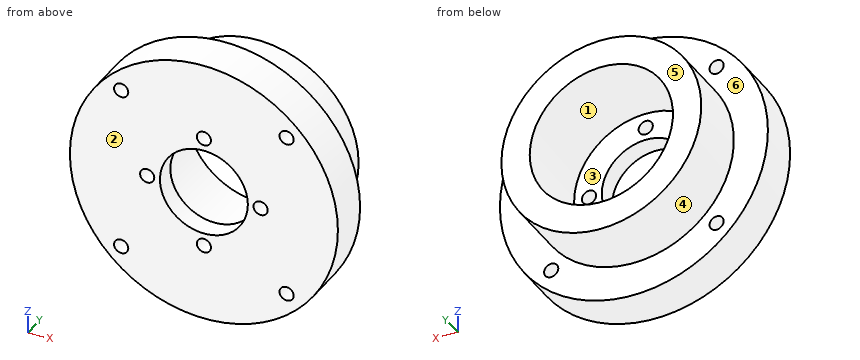
```python
from build123d import *

# Parameters (mm, degrees)
SKETCH1_R           = 35.25
SKETCH1_R_2         = 15.5
BOSS_EXTRUDE1_DEPTH = 7
SKETCH2_R           = 35.25
SKETCH2_R_2         = 25.25
BOSS_EXTRUDE2_DEPTH = 30
SKETCH3_R           = 2.5
CUT_EXTRUDE1_DEPTH  = 7
SKETCH4_R           = 47.25
SKETCH4_R_2         = 35.25
BOSS_EXTRUDE3_DEPTH = 15
SKETCH5_R           = 2.5
CUT_EXTRUDE2_DEPTH  = 15


with BuildPart() as part:
    # Sketch1 → Boss-Extrude1 (new body)
    with BuildSketch(Plane(origin=(0, 0, 0), x_dir=(1, 0, 0), z_dir=(0, 1, 0))):
        Circle(SKETCH1_R)
        Circle(SKETCH1_R_2, mode=Mode.SUBTRACT)
    extrude(amount=BOSS_EXTRUDE1_DEPTH)

    # Sketch2 → Boss-Extrude2 (add)
    with BuildSketch(Plane(origin=(0, 7, 0), x_dir=(1, 0, 0), z_dir=(0, 1, 0))):
        Circle(SKETCH2_R)
        Circle(SKETCH2_R_2, mode=Mode.SUBTRACT)
    extrude(amount=BOSS_EXTRUDE2_DEPTH)

    # Sketch3 → Cut-Extrude1 (cut)
    with BuildSketch(Plane(origin=(0, 7, 0), x_dir=(1, 0, 0), z_dir=(0, 1, 0))):
        with Locations((0, 20)):
            Circle(SKETCH3_R)
        with Locations((20, 0)):
            Circle(SKETCH3_R)
        with Locations((0, -20)):
            Circle(SKETCH3_R)
        with Locations((-20, 0)):
            Circle(SKETCH3_R)
    extrude(amount=-CUT_EXTRUDE1_DEPTH, mode=Mode.SUBTRACT)

    # Sketch4 → Boss-Extrude3 (add)
    with BuildSketch(Plane.XZ):
        Circle(SKETCH4_R)
        Circle(SKETCH4_R_2, mode=Mode.SUBTRACT)
    extrude(amount=-BOSS_EXTRUDE3_DEPTH)

    # Sketch5 → Cut-Extrude2 (cut)
    with BuildSketch(Plane.XZ):
        with Locations((29.168154724, 29.168154724)):
            Circle(SKETCH5_R)
        with Locations((29.168154724, -29.168154724)):
            Circle(SKETCH5_R)
        with Locations((-29.168154724, -29.168154724)):
            Circle(SKETCH5_R)
        with Locations((-29.168154724, 29.168154724)):
            Circle(SKETCH5_R)
    extrude(amount=-CUT_EXTRUDE2_DEPTH, mode=Mode.SUBTRACT)


solid = part.part
```
Can you work these out from the model? Positions are in its coordinate system, mm. Face numbers are marked on the shaded views. A direction names the side the tool comes from. Round coordinates to 2 decimals unless told otherwise and drop trailing zeros. Order: outer loops, then holes, each group sorted by start corner. A loop starts at its lowest first (then second) coordinate and runs counter-clockwise, first axis right, second up. Notation, with made-up numbers: (-23, 67.25) -> (13, 67.25) arc R22 ccw to (13, 87.25) -> close; hole circle Ø2 at (41, 12.5). An arc over 180 degrees is marked (long way). Return JSON: item names as keys, results as strings. Group by question number.
1. We'd pull the mould along Z, two halves only. Please class the marked faces 1, 2, 3 and 4: released by +Z, released by -Z, zero draft, split by the parting line, or undercut.
2. Which directions (+Z, -Z, +X, -X, +Y, -Y) give clear straight access to the entire face, cutting with the end or side of a thin tool? Please do the marked faces 5 and 6.
3. If we section it at C-C, the plane y = 30: Write out the boundary of the cut face in (x, z).
4. If we section it at B-B, the plane z = 7: Write out the boundary of the cut face in (x, y), then the cut area to 3 significant figures.
5. If we section it at A-A, the plane x = -20: Write out the boundary of the cut face in (y, z).
6. If we section it at D-D, the plane z = -33: Write out the boundary of the cut face in (x, y).
7. I need wall thicknesses on line 1 (Z direction, x = 0, y = 1.5); line 2 (Z direction, x = 18.5, y = 8.5); line 3 (X direction, y = 1.5, z = 20). Which ranges of each line are inside material? Lowest first, please. Write a range as [from, to].
8. Will these pins go through, and if not, where does the flat tip stop? pin 1 (12 mm diameter, centred on x = -2, z = 22.5, fed in from -Y); pin 2 (10 mm diameter, centred on x = 17.5, y = 7.5, fed in from -Z); pin 3 (10 mm diameter, centred on x = -2, y = 22.5, fed in from -Z); pin 4 (3 mm diameter, centred on x = 33, y = 5.5, fed in from +Z).
Output values:
{
 "1": {"face 1": "undercut", "face 2": "zero draft", "face 3": "undercut", "face 4": "split by the parting line"},
 "2": {"face 5": "+Z, -Z, +X, -X, +Y", "face 6": "+Y"},
 "3": {"outline": "circle Ø70.5 at (0, 0); hole circle Ø50.5 at (0, 0)"},
 "4": {"outline": "(-46.73, 0) -> (-13.83, 0) -> (-13.83, 7) -> (-24.26, 7) -> (-24.26, 37) -> (-34.55, 37) -> (-34.55, 15) -> (-46.73, 15) -> close; (13.83, 0) -> (46.73, 0) -> (46.73, 15) -> (34.55, 15) -> (34.55, 37) -> (24.26, 37) -> (24.26, 7) -> (13.83, 7) -> close", "area": "1,270 mm²"},
 "5": {"outline": "(0, -42.81) -> (15, -42.81) -> (15, -29.03) -> (37, -29.03) -> (37, -15.41) -> (7, -15.41) -> (7, -2.5) -> (0, -2.5) -> close; (0, 2.5) -> (7, 2.5) -> (7, 15.41) -> (37, 15.41) -> (37, 29.03) -> (15, 29.03) -> (15, 42.81) -> (0, 42.81) -> close"},
 "6": {"outline": "(-33.82, 0) -> (33.82, 0) -> (33.82, 15) -> (12.39, 15) -> (12.39, 37) -> (-12.39, 37) -> (-12.39, 15) -> (-33.82, 15) -> close"},
 "7": {"line 1": "[-47.25, -22.5], [-17.5, -15.5], [15.5, 17.5], [22.5, 47.25]", "line 2": "[-43.48, -17.18], [17.18, 43.48]", "line 3": "[-42.81, -2.5], [2.5, 42.81]"},
 "8": {"pin 1": "y = 0", "pin 2": "z = -45.57", "pin 3": "z = -35.25", "pin 4": "z = 35.22"}
}
